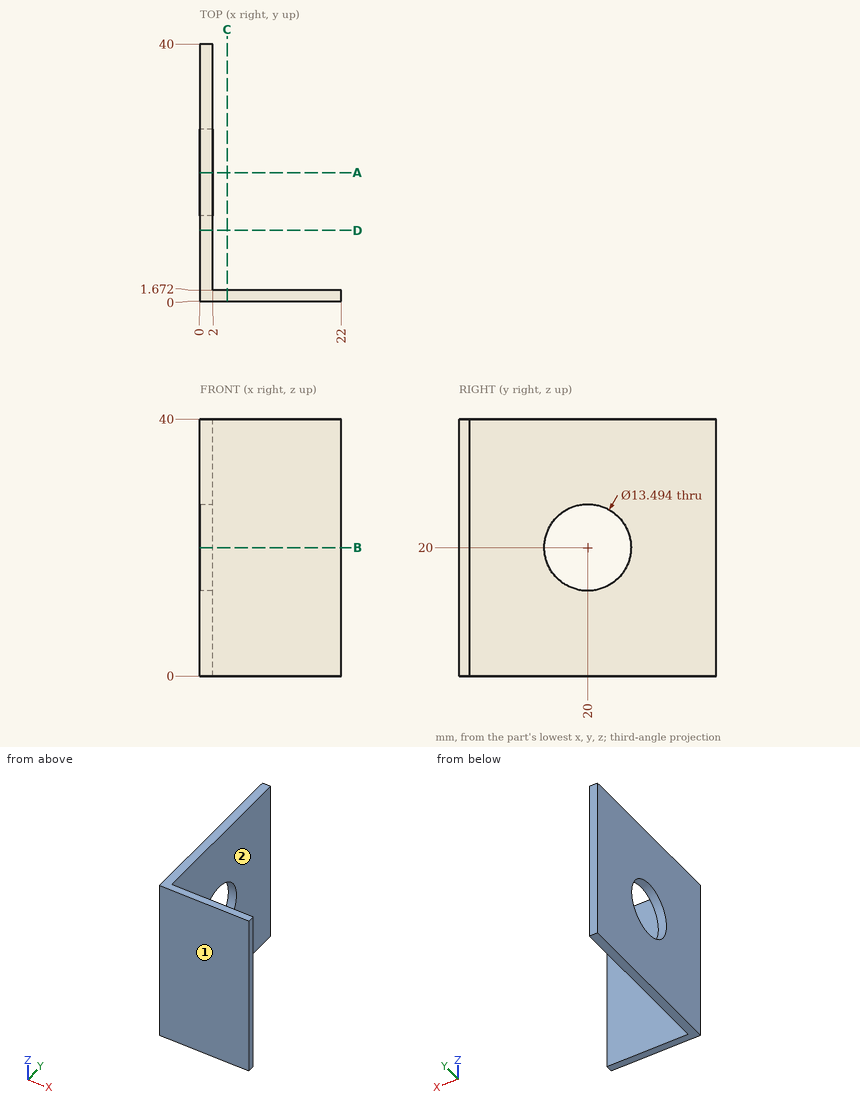
Design review of the part shown in the three views and the two pictorial views. Dimensions are in mm from the part's minimum x, y and z. A direction names the side the tool comes from. Round coordinates to 2 decimals unless told otherwise and drop trailing zeros. Loops run counter-clockwise (first coordinate to the right, second up) from the corner with the lowest first, then second, coordinate; pieces in that order, holes last. Notation, with made-up numbers: (2.25, 1) - (25.25, 1) arc R19 cw to (25.25, 15) - close; hole circle Ø7 at (-31.75, 84.25). An arc over 180 degrees is marked (long way). Write each question's results on one line, items separated by ' | '. Start each with the question number.
Q1. Take a section at D-D on y = 11. Give the boundary of the cut face in (x, z).
Q2. Take a section at A-A on y = 20. Give the boundary of the cut face in (x, z).
Q3. Take a section at B-B on z = 20. Give the boundary of the cut face in (x, y).
Q4. Tool access review of the marked faces 1 and 2: name each direction out of +Z, -Z, +X, -X, +Y, -Y from which nothing blocks a thin tool from reaching the whole face with its end or side.
Q5. Take a section at C-C on x = 4.25. Give the boundary of the cut face in (y, z).
Q6. Wall thickness on line 1 along Y through (x, z) = (0.95, 20); line 2 along Y through (x, z) = (18, 28.5); line 3 along X through (y, z) = (9.5, 20.5): over which ranges is each line inside the solid? List them lowest first. Write a range as [from, to].
Q7. Insertion check: P1, Ø5, axis at x = 13.5, z = 12, coming from the +Y side; P2, Ø10, axis at y = 19.5, z = 25, coming from the +X side. Each pin has a flat end and moves straight along its axis. Give the tip position at first contact, or say it passes through.
Data:
1) outline: (0, 0) - (2, 0) - (2, 40) - (0, 40) - close
2) outline: (0, 0) - (2, 0) - (2, 13.25) - (0, 13.25) - close; (0, 26.75) - (2, 26.75) - (2, 40) - (0, 40) - close
3) outline: (0, 0) - (22, 0) - (22, 1.67) - (2, 1.67) - (2, 13.25) - (0, 13.25) - close; (0, 26.75) - (2, 26.75) - (2, 40) - (0, 40) - close
4) face 1: +Z, -Z, +X, -X, -Y | face 2: +Z, -Z, +X, +Y
5) outline: (0, 0) - (1.67, 0) - (1.67, 40) - (0, 40) - close
6) line 1: y = [0, 13.25], [26.75, 40] | line 2: y = [0, 1.67] | line 3: x = [0, 2]
7) P1: stops at y = 1.67 | P2: stops at x = 2
